Can you work these out from the model? Positions are in its coordinate system, mm. Coordinates: 2 decimals unless noted, no trailing zeros. Write each loop counter-clockwise with the first axis right and the second up, starting at its lowest first coordinate (ties: lowest second). Pieces come first, ordered by that corner, then holes. Notation, with made-up numbers: (1.25, 61.25) -> (15.25, 61.25) arc R31 ccw to (15.25, 90.25) -> close; hole circle Ø5 at (63, -17). An arc over 180 degrees is marked (long way). Answer as CSV lines item,"result". Start each with the question number.
Autodesk Inventor part; units mm, degrees
ref_plane "Work Plane2" through (1, 0, 0) normal (1, 0, 0) x (0, 1, 0)
ref_plane "Work Plane8" through (2, 0, 0) normal (1, 0, 0) x (0, 1, 0)
ref_plane "Work Plane6" through (3, 0, 0) normal (1, 0, 0) x (0, 1, 0)
sketch "Sketch1" plane through (0, 0, 0) normal (1, 0, 0) x (0, 1, 0)
  line L0 (-28.3154, 9.9073) -> (-28.3154, -18.0927)
  line L1 (13.6846, -4.0927) -> (13.6846, -9.0927)
  line L2 (13.6846, -4.0927) -> (13.6846, 0.9073)
  line L3 (-28.3154, 9.9073) -> (13.6846, 0.9073)
  line L4 (-28.3154, -18.0927) -> (13.6846, -9.0927)
  point P0 (0, 0)
ref_plane "Work Plane2" through (1, 0, 0) normal (1, 0, 0) x (0, 1, 0)
sketch "Sketch5" plane through (1, 0, 0) normal (1, 0, 0) x (0, 1, 0)
  line L0 (-29.3154, 9.9073) -> (12.6846, 0.9073)
  line L1 (12.6846, -4.0927) -> (12.6846, 0.9073)
  line L2 (12.6846, -4.0927) -> (12.6846, -9.0927)
  line L3 (-29.3154, -18.0927) -> (12.6846, -9.0927)
  line L4 (-29.3154, 9.9073) -> (-29.3154, -18.0927)
  point P0 (0, 0)
loft "Loft1" add profiles "Sketch1", "Sketch5"
ref_plane "Work Plane8" through (2, 0, 0) normal (1, 0, 0) x (0, 1, 0)
sketch "Sketch8" plane through (2, 0, 0) normal (1, 0, 0) x (0, 1, 0)
  line L0 (-30.3154, 9.9073) -> (11.6846, 0.9073)
  line L1 (11.6846, -9.0927) -> (-30.3154, -18.0927)
  line L2 (-30.3154, -18.0927) -> (-30.3154, 9.9073)
  line L3 (11.6846, 0.9073) -> (11.6846, -9.0927)
  point P0 (0, 0)
loft "Loft2" add profiles "Sketch8" section 1 edges at (1, -29.3154, -4.0927) (1, -8.3154, -13.5927) (1, 12.6846, -6.5927) (1, 12.6846, -1.5927) (1, -8.3154, 5.4073)
ref_plane "Work Plane6" through (3, 0, 0) normal (1, 0, 0) x (0, 1, 0)
sketch "Sketch9" plane through (3, 0, 0) normal (1, 0, 0) x (0, 1, 0)
  line L0 (-31.3154, 9.9073) -> (-31.3154, -18.0927)
  line L1 (-31.3154, -18.0927) -> (10.6846, -9.0927)
  line L2 (10.6846, -9.0927) -> (10.6846, 0.9073)
  line L3 (10.6846, 0.9073) -> (-31.3154, 9.9073)
  line L4 (11.6846, -9.0927) -> (11.6846, 0.9073)
  point P0 (-1, 0)
loft "Loft3" add profiles "Sketch9" section 1 edges at (2, -30.3154, -4.0927) (2, -9.3154, -13.5927) (2, 11.6846, -4.0927) (2, -9.3154, 5.4073)
sketch "Sketch10" plane through (3, -31.3154, 9.9073) normal (1, 0, 0) x (0, 0, -1)
  circle A0 centre (5, 5.2079) radius 1
  circle A1 centre (23, 5.2079) radius 1
  circle A2 centre (14, 38.9079) radius 1
  point P0 (9.9073, 31.3154)
  dimension "d36" = 33.7
  dimension "d37" = 33.7
  dimension "d38" = 18
  dimension "d39" = 9
extrude "Extrusion1" cut sketch "Sketch10" against normal blind 3
chamfer "Chamfer1" distance 0.5 angle 45 1 edges at (3, -26.1075, 5.9073)
chamfer "Chamfer2" distance 0.5 angle 45 2 edges at (3, -26.1075, -12.0927) (3, 7.5925, -3.0927)
properties part number "triangular"
Q1. For pin 1 (1.8 mm diameter, centred on y = 7.59, z = -4.09, fed in from -X); pin 2 (1 mm diameter, centred on x = 1, z = -9.5, fed in from -Y); pin 3 (2.5 mm diameter, centred on y = -26.11, z = 4.91, fed in from +X), each with a flat end and sliding along its axis, tell me the tip position at first contact or that it passes through.
Q2. I need wall thicknesses on L1, parallel to Z at x = 1.9, y = 7; L2, parallel to Y at x = 0.1, z = -5; L3, parallel to Z at x = 1.55, y = -25.5. Which ranges of each line are inside material? Lowest first, please.
Q3. If we mould it in two halves opening along Z, with no side actions, what happens to faces 1 (the face through (0, -10, -4)), 2 (the face through (1.268, 8.584, -3.963)), 3 (the face through (1.268, -25.116, 5.037)), 4 (the face through (1.52, -9.13, 5.47))? For each: released by +Z, released by -Z, zero draft, split by the parting line, or undercut.
Q4. Imagine slicing it at C-C (y = -4). Write out the boundary of the cut face in (x, z), then the cut area to 3 significant figures.
Q5. Imagine slicing it at A-A (x = 1.75). Write out the boundary of the cut face in (y, z).
Q6. Imagine slicing it at B-B (z = -0.5). Write out the boundary of the cut face in (x, y), then the cut area to 3 significant figures.
Entries:
1,pin 1,"through"
1,pin 2,"y = -29.82"
1,pin 3,"x = 2.75"
2,L1,"-10.12 to -4.9, -3.29 to 1.93"
2,L2,"-28.42 to 7.17, 8.01 to 13.58"
2,L3,"-17.16 to -13.89, -12.3 to 4.11, 5.7 to 8.97"
3,face 1,"zero draft"
3,face 2,"undercut"
3,face 3,"undercut"
3,face 4,"released by +Z"
4,outline,"(0, -12.88) -> (3, -12.24) -> (3, 4.05) -> (0, 4.7) -> close"
4,area,"50.8 mm2"
5,outline,"(-30.07, -18.09) -> (11.93, -9.09) -> (11.93, 0.91) -> (-30.07, 9.91) -> close; hole circle Ø2 at (-26.11, -13.09); hole circle Ø2 at (-26.11, 4.91); hole circle Ø2 at (7.59, -4.09)"
6,outline,"(0, -28.32) -> (3, -31.32) -> (3, 10.68) -> (0, 13.68) -> close"
6,area,"126 mm2"
